Study the drawing (mm; zero at the part's minimum x, y, z) and answer. A direction names the side the tool comes from. Give positions to 0.01 mm unless a question says otherwise; leave off trailing zeros. Loops run counter-clockwise (first coordinate to the right, second up) from the corner with the lowest first, then second, coordinate; pieces in that order, holes last. Notation, with made-up numbers: M 85,80.5 L 134,80.5 A26 cw 134,107.5 Z; hole C 73,76 d6. An arc over 180 degrees is marked long. Return JSON: item names as keys, results as strings.
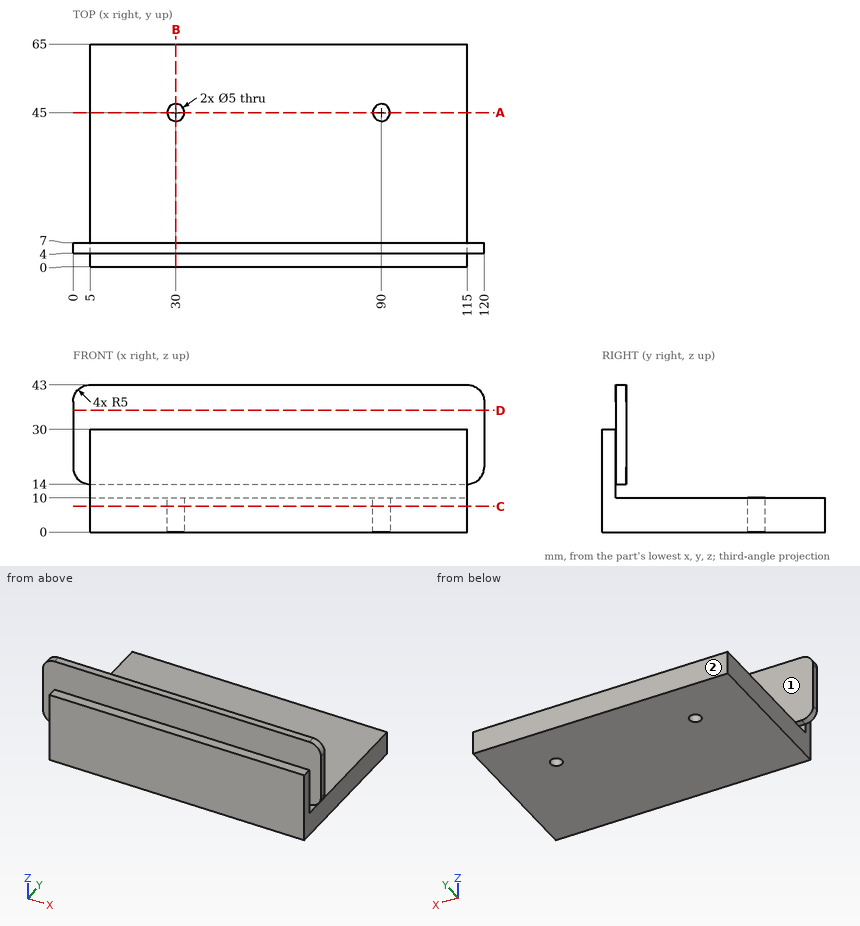
(1) Given pin 1 (9 mm diameter, centred on y = 48.5, z = 13.5, fed in from +X); pin 2 (10 mm diameter, centred on x = 22, y = 47.5, fed in from +Z); pin 3 (8.5 mm diameter, centred on x = 51, z = 26, fed in from +Y), each flat-ended and moving along its own axis, determine where each tip first touches the part or whether it passes through.
Values follow:
{"pin 1": "x = 115", "pin 2": "z = 10", "pin 3": "y = 7"}
(2) The part is cut by section C-C (z = 7.5). Determine the outline of the cut face in (x, y).
Values follow:
{"outline": "M 5,0 L 115,0 L 115,65 L 5,65 Z; hole C 30,45 d5; hole C 90,45 d5"}
(3) The part is cut by section D-D (z = 35.5). Determine the outline of the cut face in (x, y), and give its area (3 significant figures).
Values follow:
{"outline": "M 0,4 L 120,4 L 120,7 L 0,7 Z", "area": "360 mm²"}
(4) Straight lines are drawn through the part: line 1 along Y through (x, z) = (90, 4.75); line 2 along Z through (x, y) = (52.5, 10.5); line 3 along Y through (x, z) = (59, 32.5). For each, find the intervals that lie inside material, in ascending order.
Values follow:
{"line 1": "0 to 42.5, 47.5 to 65", "line 2": "0 to 10", "line 3": "4 to 7"}
(5) A tool of negligible diameter and unlimited length cuts with its end or side. For the marked faces 1 and 2, from which of +Z, -Z, +X, -X, +Y, -Y can it reach the whole face along a straight path? Write none if from no direction.
Values follow:
{"face 1": "+Z, +X, -X, +Y", "face 2": "+Z, -Z, +X, -X, +Y"}
(6) The part is cut by section B-B (x = 30). Determine the outline of the cut face in (y, z).
Values follow:
{"outline": "M 0,0 L 42.5,0 L 42.5,10 L 4,10 L 4,14 L 7,14 L 7,43 L 4,43 L 4,30 L 0,30 Z; M 47.5,0 L 65,0 L 65,10 L 47.5,10 Z"}
(7) The part is cut by section A-A (y = 45). Determine the outline of the cut face in (x, z), and give its area (3 significant figures).
Values follow:
{"outline": "M 5,0 L 27.5,0 L 27.5,10 L 5,10 Z; M 32.5,0 L 87.5,0 L 87.5,10 L 32.5,10 Z; M 92.5,0 L 115,0 L 115,10 L 92.5,10 Z", "area": "1,000 mm²"}
